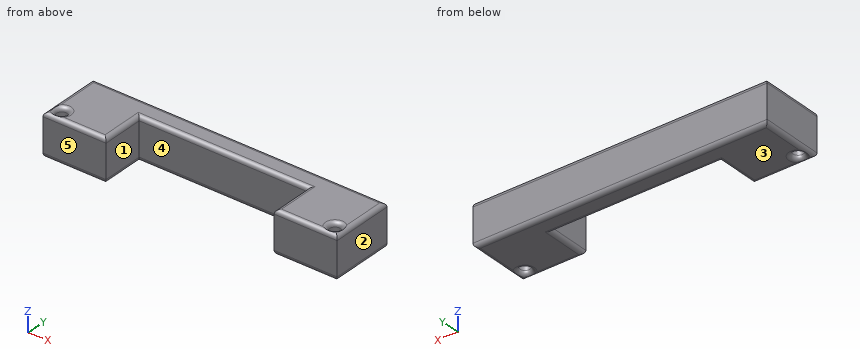
from build123d import *

# Parameters (mm, degrees)
F1_DEPTH     = 20
F3_D         = 5
F5_T1_DEPTH  = 150
F5_T3_DEPTH  = 40
F5_T5_DEPTH  = 40
F5_T7_DEPTH  = 25
F5_T9_DEPTH  = 80
F5_T11_DEPTH = 40
F5_T25_DEPTH = 85
F5_T29_DEPTH = 30
F5_T36_DEPTH = 30
F5_T40_DEPTH = 85
F5_T47_DEPTH = 30
F5_T51_DEPTH = 85
F5_T58_DEPTH = 85
F5_T62_DEPTH = 30


# Not quite as in the source:
# - a fillet or chamfer that OpenCascade refuses, or shapes differently, is made with other operations: its cross-section is extruded or revolved along the edge and cut away or added


with BuildPart() as f1:
    # F0 (on Top) → F1 (new body)
    with BuildSketch(Plane.XY):
        Polygon((70, 32.1153850414), (0, 32.1153850414), (0, 22.1153850414), (40, 22.1153850414), (40, 2.1153850414), (70, 2.1153850414), align=None)
    extrude(amount=F1_DEPTH)

    # F3 (through all)
    with Locations(Plane.XY.offset(20)):
        with Locations((65, 7.1153850414)):
            Hole(F3_D / 2)

    # F4: F1 across face


with BuildPart() as f1_1:
    add(f1.part)
    add(f1.part.mirror(Plane(origin=(0, 27.1153850414, 10), x_dir=(0, -1, 0), z_dir=(-1, 0, 0))))

    # F5: fillet of radius 2 on 20 edges, made by hand

    # F5_s2 → F5_t1 (cut)
    with BuildSketch(Plane.YZ.offset(-75)):
        with BuildLine():
            ThreePointArc((32.1153850414, 18), (31.5295986038, 19.4142135624), (30.1153850414, 20))
            Line((30.1153850414, 20), (32.1153850414, 20))
            Line((32.1153850414, 20), (32.1153850414, 18))
        make_face()
        with BuildLine():
            ThreePointArc((32.1153850414, 2), (31.5295986038, 0.5857864376), (30.1153850414, 0))
            Line((30.1153850414, 0), (32.1153850414, 0))
            Line((32.1153850414, 0), (32.1153850414, 2))
        make_face()
    extrude(amount=F5_T1_DEPTH, mode=Mode.SUBTRACT)

    # F5_s4 → F5_t3 (cut)
    with BuildSketch(Plane.XZ.offset(-37.1153850414)):
        with BuildLine():
            ThreePointArc((-70, 18), (-69.4142135624, 19.4142135624), (-68, 20))
            Line((-68, 20), (-70, 20))
            Line((-70, 20), (-70, 18))
        make_face()
        with BuildLine():
            ThreePointArc((68, 20), (69.4142135624, 19.4142135624), (70, 18))
            Line((70, 18), (70, 20))
            Line((70, 20), (68, 20))
        make_face()
        with BuildLine():
            ThreePointArc((-68, 0), (-69.4142135624, 0.5857864376), (-70, 2))
            Line((-70, 2), (-70, 0))
            Line((-70, 0), (-68, 0))
        make_face()
        with BuildLine():
            ThreePointArc((68, 0), (69.4142135624, 0.5857864376), (70, 2))
            Line((70, 2), (70, 0))
            Line((70, 0), (68, 0))
        make_face()
    extrude(amount=F5_T3_DEPTH, mode=Mode.SUBTRACT)

    # F5_s6 → F5_t5 (cut)
    with BuildSketch(Plane.YZ.offset(-75)):
        with BuildLine():
            ThreePointArc((2.1153850414, 18), (2.701171479, 19.4142135624), (4.1153850414, 20))
            Line((4.1153850414, 20), (2.1153850414, 20))
            Line((2.1153850414, 20), (2.1153850414, 18))
        make_face()
        with BuildLine():
            ThreePointArc((4.1153850414, 0), (2.701171479, 0.5857864376), (2.1153850414, 2))
            Line((2.1153850414, 2), (2.1153850414, 0))
            Line((2.1153850414, 0), (4.1153850414, 0))
        make_face()
    extrude(amount=F5_T5_DEPTH, mode=Mode.SUBTRACT)

    # F5_s8 → F5_t7 (cut)
    with BuildSketch(Plane.XZ.offset(-22.1153850414)):
        with BuildLine():
            ThreePointArc((-40, 18), (-40.5857864376, 19.4142135624), (-42, 20))
            Line((-42, 20), (-40, 20))
            Line((-40, 20), (-40, 18))
        make_face()
        with BuildLine():
            ThreePointArc((40, 18), (40.5857864376, 19.4142135624), (42, 20))
            Line((42, 20), (40, 20))
            Line((40, 20), (40, 18))
        make_face()
        with BuildLine():
            ThreePointArc((-42, 0), (-40.5857864376, 0.5857864376), (-40, 2))
            Line((-40, 2), (-40, 0))
            Line((-40, 0), (-42, 0))
        make_face()
        with BuildLine():
            ThreePointArc((42, 0), (40.5857864376, 0.5857864376), (40, 2))
            Line((40, 2), (40, 0))
            Line((40, 0), (42, 0))
        make_face()
    extrude(amount=F5_T7_DEPTH, mode=Mode.SUBTRACT)

    # F5_s10 → F5_t9 (cut)
    with BuildSketch(Plane.YZ.offset(-40)):
        with BuildLine():
            ThreePointArc((22.1153850414, 18), (22.701171479, 19.4142135624), (24.1153850414, 20))
            Line((24.1153850414, 20), (22.1153850414, 20))
            Line((22.1153850414, 20), (22.1153850414, 18))
        make_face()
        with BuildLine():
            ThreePointArc((24.1153850414, 0), (22.701171479, 0.5857864376), (22.1153850414, 2))
            Line((22.1153850414, 2), (22.1153850414, 0))
            Line((22.1153850414, 0), (24.1153850414, 0))
        make_face()
    extrude(amount=F5_T9_DEPTH, mode=Mode.SUBTRACT)

    # F5_s12 → F5_t11 (cut)
    with BuildSketch(Plane.YZ.offset(35)):
        with BuildLine():
            ThreePointArc((2.1153850414, 18), (2.701171479, 19.4142135624), (4.1153850414, 20))
            Line((4.1153850414, 20), (2.1153850414, 20))
            Line((2.1153850414, 20), (2.1153850414, 18))
        make_face()
        with BuildLine():
            ThreePointArc((4.1153850414, 0), (2.701171479, 0.5857864376), (2.1153850414, 2))
            Line((2.1153850414, 2), (2.1153850414, 0))
            Line((2.1153850414, 0), (4.1153850414, 0))
        make_face()
    extrude(amount=F5_T11_DEPTH, mode=Mode.SUBTRACT)

    # F5_s13 → F5_t14 (revolve, cut)
    with BuildSketch(Plane.XZ.offset(-7.1153850414)):
        with BuildLine():
            ThreePointArc((67.5, 18), (68.0857864376, 19.4142135624), (69.5, 20))
            Line((69.5, 20), (67.5, 20))
            Line((67.5, 20), (67.5, 18))
        make_face()
    revolve(axis=Axis((65, 7.1153850414, 20), (0, 0, 1)), mode=Mode.SUBTRACT)

    # F5_s15 → F5_t16 (revolve, cut)
    with BuildSketch(Plane.XZ.offset(-7.1153850414)):
        with BuildLine():
            ThreePointArc((-67.5, 18), (-68.0857864376, 19.4142135624), (-69.5, 20))
            Line((-69.5, 20), (-67.5, 20))
            Line((-67.5, 20), (-67.5, 18))
        make_face()
    revolve(axis=Axis((-65, 7.1153850414, 20), (0, 0, -1)), mode=Mode.SUBTRACT)

    # F5_s17 → F5_t18 (revolve, cut)
    with BuildSketch(Plane.XZ.offset(-7.1153850414)):
        with BuildLine():
            ThreePointArc((69.5, 0), (68.0857864376, 0.5857864376), (67.5, 2))
            Line((67.5, 2), (67.5, 0))
            Line((67.5, 0), (69.5, 0))
        make_face()
    revolve(axis=Axis((65, 7.1153850414, 0), (0, 0, 1)), mode=Mode.SUBTRACT)

    # F5_s19 → F5_t20 (revolve, cut)
    with BuildSketch(Plane.XZ.offset(-7.1153850414)):
        with BuildLine():
            ThreePointArc((-69.5, 0), (-68.0857864376, 0.5857864376), (-67.5, 2))
            Line((-67.5, 2), (-67.5, 0))
            Line((-67.5, 0), (-69.5, 0))
        make_face()
    revolve(axis=Axis((-65, 7.1153850414, 0), (0, 0, -1)), mode=Mode.SUBTRACT)


with BuildPart() as f5_tool23:
    # F5_s24 → F5_t25 (new body)
    with BuildSketch(Plane.YZ.offset(-45)):
        with BuildLine():
            ThreePointArc((22.1153850414, 18), (22.701171479, 19.4142135624), (24.1153850414, 20))
            Line((24.1153850414, 20), (22.1153850414, 20))
            Line((22.1153850414, 20), (22.1153850414, 18))
        make_face()
    extrude(amount=F5_T25_DEPTH)

    split(bisect_by=Plane.YZ.offset(-40), keep=Keep.BOTTOM)


with BuildPart() as f5_tool27:
    # F5_s28 → F5_t29 (new body)
    with BuildSketch(Plane.XZ.offset(-27.1153850414)):
        with BuildLine():
            ThreePointArc((-40, 18), (-40.5857864376, 19.4142135624), (-42, 20))
            Line((-42, 20), (-40, 20))
            Line((-40, 20), (-40, 18))
        make_face()
    extrude(amount=F5_T29_DEPTH)

    split(bisect_by=Plane.XZ.offset(-22.1153850414), keep=Keep.BOTTOM)


with BuildPart() as f5_tool23_1:
    add(f5_tool23.part)

    # F5_t31: intersect F5_tool27
    add(f5_tool27.part, mode=Mode.INTERSECT)


with BuildPart() as f1_2:
    add(f1_1.part)

    # F5_t21: cut F5_tool23
    add(f5_tool23_1.part, mode=Mode.SUBTRACT)


with BuildPart() as f5_tool34:
    # F5_s35 → F5_t36 (new body)
    with BuildSketch(Plane.XZ.offset(-27.1153850414)):
        with BuildLine():
            ThreePointArc((40, 18), (40.5857864376, 19.4142135624), (42, 20))
            Line((42, 20), (40, 20))
            Line((40, 20), (40, 18))
        make_face()
    extrude(amount=F5_T36_DEPTH)

    split(bisect_by=Plane.XZ.offset(-22.1153850414), keep=Keep.BOTTOM)


with BuildPart() as f5_tool38:
    # F5_s39 → F5_t40 (new body)
    with BuildSketch(Plane.YZ.offset(-40)):
        with BuildLine():
            ThreePointArc((22.1153850414, 18), (22.701171479, 19.4142135624), (24.1153850414, 20))
            Line((24.1153850414, 20), (22.1153850414, 20))
            Line((22.1153850414, 20), (22.1153850414, 18))
        make_face()
    extrude(amount=F5_T40_DEPTH)

    split(bisect_by=Plane.YZ.offset(40), keep=Keep.TOP)


with BuildPart() as f5_tool34_1:
    add(f5_tool34.part)

    # F5_t42: intersect F5_tool38
    add(f5_tool38.part, mode=Mode.INTERSECT)


with BuildPart() as f1_3:
    add(f1_2.part)

    # F5_t32: cut F5_tool34
    add(f5_tool34_1.part, mode=Mode.SUBTRACT)


with BuildPart() as f5_tool45:
    # F5_s46 → F5_t47 (new body)
    with BuildSketch(Plane.XZ.offset(-27.1153850414)):
        with BuildLine():
            ThreePointArc((-42, 0), (-40.5857864376, 0.5857864376), (-40, 2))
            Line((-40, 2), (-40, 0))
            Line((-40, 0), (-42, 0))
        make_face()
    extrude(amount=F5_T47_DEPTH)

    split(bisect_by=Plane.XZ.offset(-22.1153850414), keep=Keep.BOTTOM)


with BuildPart() as f5_tool49:
    # F5_s50 → F5_t51 (new body)
    with BuildSketch(Plane.YZ.offset(40)):
        with BuildLine():
            ThreePointArc((24.1153850414, 0), (22.701171479, 0.5857864376), (22.1153850414, 2))
            Line((22.1153850414, 2), (22.1153850414, 0))
            Line((22.1153850414, 0), (24.1153850414, 0))
        make_face()
    extrude(amount=-F5_T51_DEPTH)

    split(bisect_by=Plane.YZ.offset(-40), keep=Keep.BOTTOM)


with BuildPart() as f5_tool45_1:
    add(f5_tool45.part)

    # F5_t53: intersect F5_tool49
    add(f5_tool49.part, mode=Mode.INTERSECT)


with BuildPart() as f1_4:
    add(f1_3.part)

    # F5_t43: cut F5_tool45
    add(f5_tool45_1.part, mode=Mode.SUBTRACT)


with BuildPart() as f5_tool56:
    # F5_s57 → F5_t58 (new body)
    with BuildSketch(Plane.YZ.offset(45)):
        with BuildLine():
            ThreePointArc((24.1153850414, 0), (22.701171479, 0.5857864376), (22.1153850414, 2))
            Line((22.1153850414, 2), (22.1153850414, 0))
            Line((22.1153850414, 0), (24.1153850414, 0))
        make_face()
    extrude(amount=-F5_T58_DEPTH)

    split(bisect_by=Plane.YZ.offset(40), keep=Keep.TOP)


with BuildPart() as f5_tool60:
    # F5_s61 → F5_t62 (new body)
    with BuildSketch(Plane.XZ.offset(-27.1153850414)):
        with BuildLine():
            ThreePointArc((42, 0), (40.5857864376, 0.5857864376), (40, 2))
            Line((40, 2), (40, 0))
            Line((40, 0), (42, 0))
        make_face()
    extrude(amount=F5_T62_DEPTH)

    split(bisect_by=Plane.XZ.offset(-22.1153850414), keep=Keep.BOTTOM)


with BuildPart() as f5_tool56_1:
    add(f5_tool56.part)

    # F5_t64: intersect F5_tool60
    add(f5_tool60.part, mode=Mode.INTERSECT)


with BuildPart() as f1_5:
    add(f1_4.part)

    # F5_t54: cut F5_tool56
    add(f5_tool56_1.part, mode=Mode.SUBTRACT)


solid = f1_5.part
Verification items for the finished model (mm, model axes). Face numbers are marked on the shaded views. A direction names the side the tool comes from. Give positions to 0.01 mm unless a question says otherwise; leave off trailing zeros. Order: outer loops, then holes, each group sorted by start corner. A loop starts at its lowest first (then second) coordinate and runs counter-clockwise, first axis right, second up. Notation, with made-up numbers: M -39.75,-4.5 L -10.75,-4.5 A12 cw -10.75,6.5 Z; hole C 56,56 d7. An arc over 180 degrees is marked long. Answer as a JSON object with one key per item and string values. Group by question number.
1) Mould release check, pull along X, two halves, no side actions. Record for the marked faces 1, 2 and 3: released by +X, released by -X, zero draft, split by the parting line, or undercut.
2) Depth check by flat-ended pin: pin 1 Ø10 at (x, z) = (-24.5, 7) entering from -Y; pin 2 Ø10 at (x, y) = (-36.5, 12.5) entering from -Z. Enter the tip coordinate at first touch or a pass-through.
3) Scan lines: line 1 along Y through (x, z) = (-65, 12); line 2 along X through (y, z) = (5.5, 8.5); line 3 along X through (y, z) = (8, 12.75). Record each from-to range of solid material in increasing order. Write a range as [from, to].
4) Cross-section at C-C (z = 13). Enter the section's corners in (x, y).
5) Cross-section at B-B (y = 15). Enter the section's corners in (x, z).
6) Access from +Z, -Z, +X, -X, +Y, -Y to the whole of each face (thin tool, end or side, straight path). Record for the marked faces 4 and 5.
7) Cross-section at A-A (x = 65). Enter the section's corners in (y, z).
8) Cross-section at D-D (x = -23). Enter the section's corners in (y, z).
Result sheet:
{
 "1": {"face 1": "undercut", "face 2": "released by +X", "face 3": "zero draft"},
 "2": {"pin 1": "stops at y = 22.12", "pin 2": "stops at z = 0.06"},
 "3": {"line 1": "y = [2.12, 4.62], [9.62, 32.12]", "line 2": "x = [-70, -66.91], [-63.09, -40], [40, 63.09], [66.91, 70]", "line 3": "x = [-70, -67.34], [-62.66, -40], [40, 62.66], [67.34, 70]"},
 "4": {"outline": "M -70,2.12 L -40,2.12 L -40,22.12 L 40,22.12 L 40,2.12 L 70,2.12 L 70,32.12 L -70,32.12 Z; hole C -65,7.12 d5; hole C 65,7.12 d5"},
 "5": {"outline": "M -70,2 A2 ccw -68,0 L -42,0 A2 ccw -40,2 L -40,18 A2 ccw -42,20 L -68,20 A2 ccw -70,18 Z; M 40,2 A2 ccw 42,0 L 68,0 A2 ccw 70,2 L 70,18 A2 ccw 68,20 L 42,20 A2 ccw 40,18 Z"},
 "6": {"face 4": "+Z, -Z, -Y", "face 5": "+Z, -Z, +X, -X, -Y"},
 "7": {"outline": "M 2.12,2 A2 ccw 3.37,0.15 A2 ccw 4.62,2 L 4.62,18 A2 ccw 3.37,19.85 A2 ccw 2.12,18 Z; M 9.62,2 A2 ccw 11.62,0 L 30.12,0 A2 ccw 32.12,2 L 32.12,18 A2 ccw 30.12,20 L 11.62,20 A2 ccw 9.62,18 Z"},
 "8": {"outline": "M 22.12,2 A2 ccw 24.12,0 L 30.12,0 A2 ccw 32.12,2 L 32.12,18 A2 ccw 30.12,20 L 24.12,20 A2 ccw 22.12,18 Z"}
}
